Check sheet for the modelled part. Datum: model origin and axes. Units: mm. Round coordinates to 2 decimals unless told otherwise and drop trailing zeros. Loops run counter-clockwise (first coordinate to the right, second up) from the corner with the lowest first, then second, coordinate; pieces in that order, holes last. Notation, with made-up numbers: (-29.5, 82.25) -> (-25.5, 82.25) arc R6 ccw to (-25.5, 91.25) -> close; hole circle Ø9 at (-5, -10). An arc over 180 degrees is marked (long way). Use one line per item in the form item = value. Start each with the question number.
(1) Material ranges on probe 1 along X at (y, z) = (-40.5, 1.4); probe 2 along X at (y, z) = (4.5, 1); probe 3 along Y at (x, z) = (-2, 2.65), recorded low to high. Write a range as [from, to].
(2) Sectioned sample at D-D (x = 4.5). Record the cut outline in (y, z) (3 decimals).
(3) Sectioned sample at A-A (z = 2.2). Record the cut outline in (x, y), and give its area (3 significant figures).
(4) Sectioned sample at C-C (y = 69). Record the cut outline in (x, z) (3 decimals).
(5) Sectioned sample at B-B (y = -4). Record the cut outline in (x, z) (3 decimals).
(6) Draft check along X on faces 1 (the cylindrical face through (-2.397, -20.074, 1.565)), 2 (the flat face through (2, -58, 3.175)). Enter one of: released by +X, released by -X, zero draft, split by the parting line, or undercut.
from build123d import *

# Parameters (mm, degrees)
BOSS_EXTRUDE1_DEPTH = 3.175
SKETCH2_W           = 3.175
SKETCH2_H           = 15
CUT_EXTRUDE1_DEPTH  = 3.175


with BuildPart() as part:
    # Sketch1 → Boss-Extrude1 (new body)
    with BuildSketch(Plane.XY):
        with BuildLine():
            ThreePointArc((-109, 88.9), (0, -20.1), (109, 88.9))
            Line((109, 88.9), (109, -88.9))
            Line((109, -88.9), (-109, -88.9))
            Line((-109, -88.9), (-109, 88.9))
        make_face()
    extrude(amount=BOSS_EXTRUDE1_DEPTH)

    # Sketch2 → Cut-Extrude1 (cut)
    with BuildSketch(Plane(origin=(0, 0, 0), x_dir=(-1, 0, 0), z_dir=(0, 0, -1))):
        with Locations((0, -44.45)):
            Rectangle(SKETCH2_W, SKETCH2_H)
    extrude(amount=-CUT_EXTRUDE1_DEPTH, mode=Mode.SUBTRACT)


solid = part.part
Checks:
q1.probe_1 = [-109, -1.59], [1.59, 109]
q1.probe_2 = [-109, -68.98], [68.98, 109]
q1.probe_3 = [-88.9, -20.08]
q2.outline = (-88.9, 0) -> (-20.007, 0) -> (-20.007, 3.175) -> (-88.9, 3.175) -> close
q3.outline = (-109, -88.9) -> (109, -88.9) -> (109, 88.9) arc R109 cw to (-109, 88.9) -> close; hole (-1.59, -51.95) -> (1.59, -51.95) -> (1.59, -36.95) -> (-1.59, -36.95) -> close
q3.area = 20,100 mm2
q4.outline = (-109, 0) -> (-107.168, 0) -> (-107.168, 3.175) -> (-109, 3.175) -> close; (107.168, 0) -> (109, 0) -> (109, 3.175) -> (107.168, 3.175) -> close
q5.outline = (-109, 0) -> (-57.014, 0) -> (-57.014, 3.175) -> (-109, 3.175) -> close; (57.014, 0) -> (109, 0) -> (109, 3.175) -> (57.014, 3.175) -> close
q6.face_1 = undercut
q6.face_2 = zero draft
